Geometry: see drawing. Coordinates: mm, zero at the bounding-box minimum. A direction names the side the tool comes from. Round coordinates to 2 decimals unless told otherwise and drop trailing zeros. Write each loop counter-clockwise with the first axis right and the second up, starting at its lowest first coordinate (ties: lowest second). Pieces come first, ordered by that corner, then holes. Notation, with made-up numbers: M 33.25,8 L 72.25,8 A20 cw 72.25,30 Z; hole C 20.25,-16 d6. An arc over 180 degrees is marked long. Use a Markdown table: item, result.
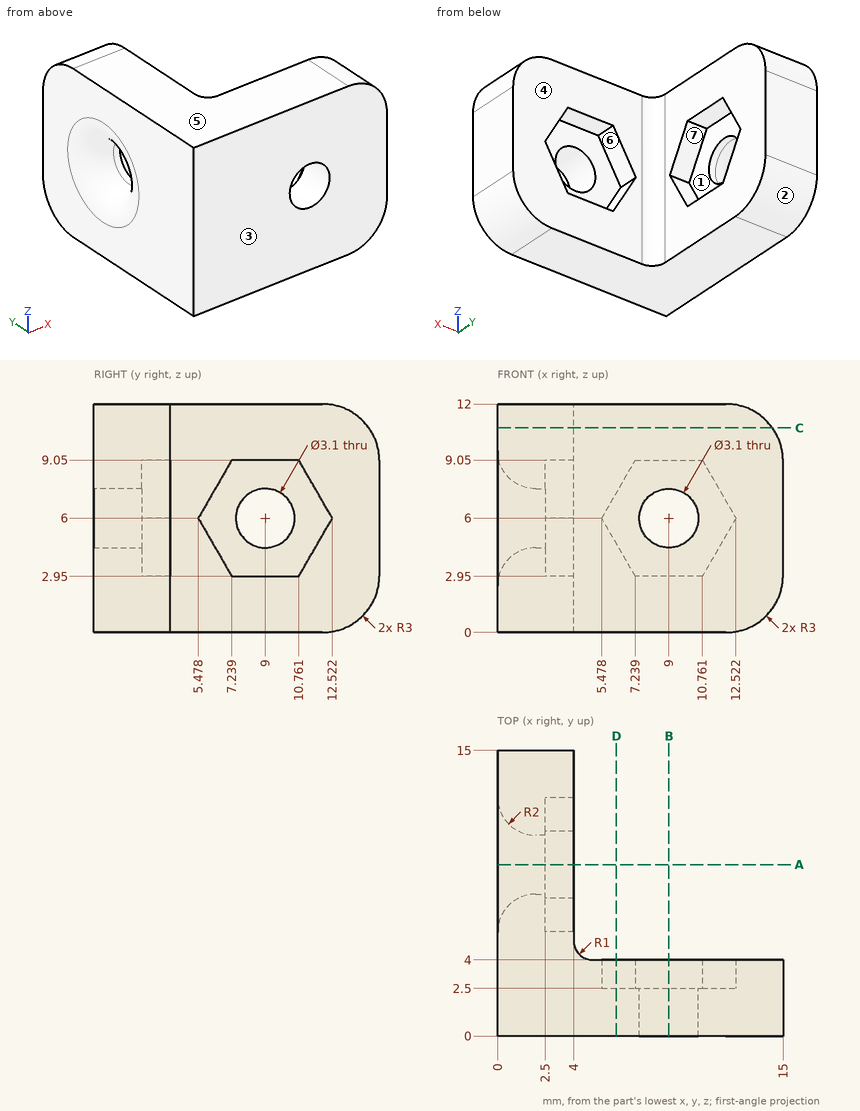
Q1. First-contact query: pin 1 Ø4 at (y, z) = (6, 2) entering from -X; pin 2 Ø6.5 at (y, z) = (8, 6) entering from +X; pin 3 Ø5 at (x, z) = (10, 9) entering from +Y; pin 4 Ø3 at (x, z) = (8.5, 6) entering from +Y. Flat tips, straight axial feed; report the tip coordinate or a pass-through.
Results are:
| item | result |
|---|---|
| pin 1 | x = 0 |
| pin 2 | x = 4.03 |
| pin 3 | y = 4 |
| pin 4 | y = 2.5 |
Q2. Section C-C on z = 10.75. Return loops of the section in (x, y).
Results are:
| item | result |
|---|---|
| outline | M 0,0 L 14.44,0 L 14.44,4 L 5,4 A1 cw 4,5 L 4,14.44 L 0,14.44 Z |
Q3. Reachability of the marked faces 4, 5, 6 and 7 from +Z, -Z, +X, -X, +Y, -Y: full face, straight path, thin tool, end or side. Return the list, or none.
Results are:
| item | result |
|---|---|
| face 4 | +Z, -Z, +X, +Y |
| face 5 | +Z, +X, -X, +Y, -Y |
| face 6 | +Y |
| face 7 | +X |
Q4. Section B-B on x = 9. Return loops of the section in (y, z), plus the area to 3 significant figures.
Results are:
| item | result |
|---|---|
| outline | M 0,0 L 4,0 L 4,2.95 L 2.5,2.95 L 2.5,4.45 L 0,4.45 Z; M 0,7.55 L 2.5,7.55 L 2.5,9.05 L 4,9.05 L 4,12 L 0,12 Z |
| area | 31.1 mm^2 |
Q5. Section A-A on y = 9. Return loops of the section in (x, z).
Results are:
| item | result |
|---|---|
| outline | M 0,0 L 4,0 L 4,2.95 L 2.5,2.95 L 2.5,4.45 L 2,4.45 A2 ccw 0,2.45 Z; M 0,9.55 A2 ccw 2,7.55 L 2.5,7.55 L 2.5,9.05 L 4,9.05 L 4,12 L 0,12 Z |
Q6. Section D-D on x = 6.25. Return loops of the section in (y, z), plus the area to 3 significant figures.
Results are:
| item | result |
|---|---|
| outline | M 0,0 L 4,0 L 4,4.66 L 2.5,4.66 L 2.5,7.34 L 4,7.34 L 4,12 L 0,12 Z |
| area | 44.0 mm^2 |
Q7. Mould query, pull axis Z, two halves, no side actions, for the marked faces 1, 2 and 3. Classes: +Z half, -Z half, draft (parallel to the pull), parting line (faces both ways), or undercut.
Results are:
| item | result |
|---|---|
| face 1 | undercut |
| face 2 | -Z half |
| face 3 | draft |
Q8. Line query: L1, parallel to X at y = 1.1, z = 6; L2, parallel to Z at x = 2.4, y = 9; L3, parallel to X at y = 5.75, z = 10. Output: solid intervals per line, ascending.
Results are:
| item | result |
|---|---|
| L1 | 0 to 7.45, 10.55 to 15 |
| L2 | 0 to 4.45, 7.55 to 12 |
| L3 | 0 to 4 |
